from build123d import *

# Parameters (mm, degrees)
F0_W      = 59.4193041325
F0_H      = 32.8746140003
F1_DEPTH  = 50
F1_FACE_W = 59.4193041325
F1_FACE_H = 50
F2_DEPTH  = 63.5828971863
F2_TAPER  = -3.0006


with BuildPart() as f1:
    # F0 (on Top) → F1 (new body)
    with BuildSketch(Plane.XY):
        with Locations((29.7096520662, -16.4373070002)):
            Rectangle(F0_W, F0_H)
    extrude(amount=F1_DEPTH)

    # F1_face (on face) → F2 (join)
    with BuildSketch(Plane(origin=(29.7096520662, -32.8746140003, 25), x_dir=(1, 0, 0), z_dir=(0, -1, 0))):
        Rectangle(F1_FACE_W, F1_FACE_H)
    extrude(amount=F2_DEPTH, taper=F2_TAPER)


solid = f1.part
Input: part model. Units: mm. Frame: model coordinates. A direction names the side the tool comes from. Coordinates: 2 decimals unless noted, no trailing zeros. Write each loop counter-clockwise with the first axis right and the second up, starting at its lowest first coordinate (ties: lowest second). Pieces come first, ordered by that corner, then holes. Notation, with made-up numbers: M 22.5,-4 L 27.5,-4 A26 ccw 27.5,12 Z; hole C 19.5,2.5 d11. An arc over 180 degrees is marked long. Answer as a JSON object with one key per item and string values. Group by question number.
(1) Set-up query: faces 1 (the face through (0, -17, 25)), 2 (the face through (29, -16, 50)), 3 (the face through (59.419, -17, 25)). Return all of +Z, -Z, +X, -X, +Y, -Y with unobstructed straight access to the full face (end or side cutting, diameter ignored); none if empty.
(2) Section A-A on y = -18.5. Output: boundary loops of the cut face in (x, z).
(3) Ray query, line 1 along Z through (x, y) = (36.5, -31); line 2 along X through (y, z) = (-6, 43.5); line 3 along X through (y, z) = (-37, 46). Return the intervals inside material, ascending. Write a range as [from, to].
(4) Contact query for flat-ended pins moving along their axis: P1, Ø10, axis at y = -43, z = 9.5, coming from the +X side; P2, Ø6, axis at x = 46, y = -43, coming from the -Z side; P3, Ø1.5, axis at y = -63.5, z = 33.5, coming from the +X side. Output: stop coordinate, or through.
Result set:
{
 "1": {"face 1": "+Z, -Z, -X, +Y", "face 2": "+Z, +X, -X, +Y", "face 3": "+Z, -Z, +X, +Y"},
 "2": {"outline": "M 0,0 L 59.42,0 L 59.42,50 L 0,50 Z"},
 "3": {"line 1": "z = [0, 50]", "line 2": "x = [0, 59.42]", "line 3": "x = [-0.22, 59.64]"},
 "4": {"P1": "stops at x = 60.21", "P2": "stops at z = -0.69", "P3": "stops at x = 61.06"}
}
